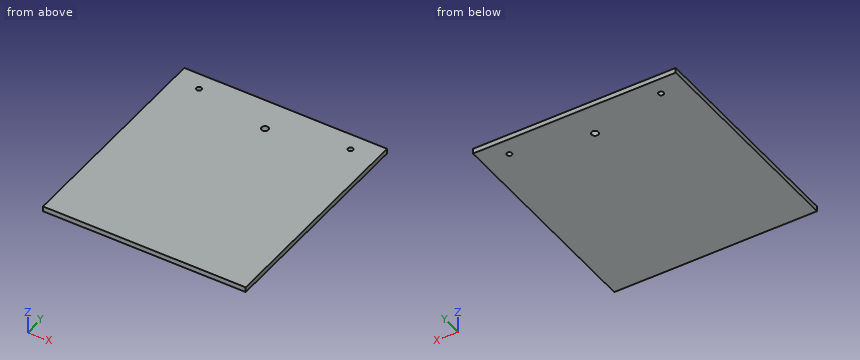
```python
from build123d import *

# Parameters (mm, degrees)
SKETCH_1_W          = 119
SKETCH_1_H          = 130
EXTRUDE_1_DEPTH     = 3
SKETCH_2_R          = 1.5
CUT_EXTRUDE_1_DEPTH = 89.17170748
SKETCH_4_R          = 2
CUT_EXTRUDE_2_DEPTH = 89.17170748


with BuildPart() as part:
    # 草图1 → 凸台-拉伸1 (new body)
    with BuildSketch(Plane.XY):
        Rectangle(SKETCH_1_W, SKETCH_1_H)
    extrude(amount=EXTRUDE_1_DEPTH)

    # 草图2 → 切除-拉伸1 (cut, through all)
    with BuildSketch(Plane.XY.offset(3)):
        with Locations((44.5, 55)):
            Circle(SKETCH_2_R)
        with Locations(Location((-44.5, 55, 0), (0, 0, 180))):
            Circle(SKETCH_2_R)
    extrude(amount=-CUT_EXTRUDE_1_DEPTH, mode=Mode.SUBTRACT)

    # 草图4 → 切除-拉伸2 (cut, through all)
    with BuildSketch(Plane.XY.offset(3)):
        with Locations((0, 46)):
            Circle(SKETCH_4_R)
    extrude(amount=-CUT_EXTRUDE_2_DEPTH, mode=Mode.SUBTRACT)


solid = part.part
```
Check sheet for the modelled part. Datum: model origin and axes. Units: mm. Give positions to 0.01 mm unless a question says otherwise; leave off trailing zeros. Write each loop counter-clockwise with the first axis right and the second up, starting at its lowest first coordinate (ties: lowest second). Pieces come first, ordered by that corner, then holes. Notation, with made-up numbers: (62.5, 67) - (111.5, 67) arc R19 cw to (111.5, 81) - close; hole circle Ø5 at (-16.5, 85.5). An arc over 180 degrees is marked (long way). Answer as a JSON object with one key per item and string values. Group by question number.
1) Thickness scan on probe 1 along Y at (x, z) = (-45.5, 0.6). Record the ranges inside material, lowest first. Write a range as from..to.
2) Sectioned sample at C-C (x = 44.5). Record the cut outline in (y, z).
3) Sectioned sample at B-B (x = 0). Record the cut outline in (y, z), then the cut area to 3 significant figures.
4) Sectioned sample at A-A (y = 55). Record the cut outline in (x, z), then the cut area to 3 significant figures.
Geometry results:
{
 "1": {"probe 1": "y = -65..53.88, 56.12..65"},
 "2": {"outline": "(-65, 0) - (53.5, 0) - (53.5, 3) - (-65, 3) - close; (56.5, 0) - (65, 0) - (65, 3) - (56.5, 3) - close"},
 "3": {"outline": "(-65, 0) - (44, 0) - (44, 3) - (-65, 3) - close; (48, 0) - (65, 0) - (65, 3) - (48, 3) - close", "area": "378 mm^2"},
 "4": {"outline": "(-59.5, 0) - (-46, 0) - (-46, 3) - (-59.5, 3) - close; (-43, 0) - (43, 0) - (43, 3) - (-43, 3) - close; (46, 0) - (59.5, 0) - (59.5, 3) - (46, 3) - close", "area": "339 mm^2"}
}
